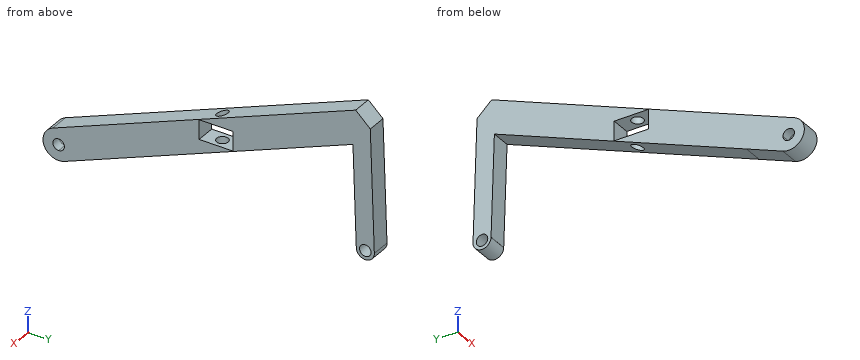
```python
from build123d import *

# Parameters (mm, degrees)
BOSS_EXTRUDE1_DEPTH     = 2.54
SKETCH2_W               = 5.08
SKETCH2_H               = 8.89
CUT_EXTRUDE1_DEPTH      = 5.08
CUT_EXTRUDE2_DEPTH      = 86.150645665
CUT_EXTRUDE2_DEPTH_BACK = 86.150645665
SKETCH3_R               = 1.5


with BuildPart() as part:
    # Sketch1 → Boss-Extrude1 (new, symmetric)
    with BuildSketch(Plane(origin=(0, 0, 0), x_dir=(0, 0, -1), z_dir=(1, 0, 0))):
        with BuildLine():
            ThreePointArc((-3.792924612, -1.516297351), (1.516297351, -3.792924612), (3.792924612, 1.516297351))
            Line((3.792924612, 1.516297351), (0, 11.004065103))
            Line((0, 11.004065103), (-26.293066659, 76.774555024))
            Line((-26.293066659, 76.774555024), (0, 77.645444775))
            Line((0, 77.645444775), (0, 77.657240774))
            Line((0, 77.657240774), (0.077903078, 77.648025113))
            ThreePointArc((0.077903078, 77.648025113), (2.351974887, 80.077903078), (-0.077903078, 82.351974887))
            Line((-0.077903078, 82.351974887), (-31.810501027, 81.300914746))
            Line((-31.810501027, 81.300914746), (-35.377927791, 77.491646464))
            Line((-35.377927791, 77.491646464), (-3.792924612, -1.516297351))
        make_face()
        with BuildLine():
            ThreePointArc((1.5, 0), (-1.060660172, -1.060660172), (0, 1.5))
            ThreePointArc((0, 1.5), (1.060660172, 1.060660172), (1.5, 0))
        make_face(mode=Mode.SUBTRACT)
        with BuildLine():
            ThreePointArc((1.5, 80), (1.060660172, 78.939339828), (0, 78.5))
            ThreePointArc((0, 78.5), (-1.060660172, 81.060660172), (1.5, 80))
        make_face(mode=Mode.SUBTRACT)
    extrude(amount=BOSS_EXTRUDE1_DEPTH, both=True)

    # Sketch2 → Cut-Extrude1 (cut)
    with BuildSketch(Plane(origin=(2.54, 0, 0), x_dir=(0, 0, -1), z_dir=(1, 0, 0))):
        with Locations((-16.420936138, 41.075962298)):
            Rectangle(SKETCH2_W, SKETCH2_H)
    extrude(amount=-CUT_EXTRUDE1_DEPTH, mode=Mode.SUBTRACT)

    # Sketch3 → Cut-Extrude2 (cut, two sides: drawn at the far end of the back side and taken through both)
    with BuildSketch(Plane.XY.offset(13.880936138).offset(-CUT_EXTRUDE2_DEPTH_BACK)):
        with Locations(Location((0, 41.075962298, 0), (0, 0, 90))):
            Circle(SKETCH3_R)
    extrude(amount=CUT_EXTRUDE2_DEPTH + CUT_EXTRUDE2_DEPTH_BACK, mode=Mode.SUBTRACT)


solid = part.part
```
Input: part model. Units: mm. Frame: model coordinates. Round coordinates to 2 decimals unless told otherwise and drop trailing zeros. Loops run counter-clockwise (first coordinate to the right, second up) from the corner with the lowest first, then second, coordinate; pieces in that order, holes last. Notation, with made-up numbers: (20, -16) -> (67, -16) arc R23 ccw to (67, -2) -> close; hole circle Ø8 at (-29.5, 61). An arc over 180 degrees is marked (long way). Use one line per item in the form item = value. Start each with the question number.
Item 1: Contact query for flat-ended pins moving along their axis: pin 1 Ø1.5 at (x, z) = (-1.5, 26.5) entering from +Y; pin 2 Ø2.5 at (x, z) = (-0.5, 17) entering from +Y; pin 3 Ø1.5 at (x, y) = (0, 40) entering from +Z; pin 4 Ø4 at (y, z) = (0, 0) entering from +X. Output: stop coordinate, or through.
Item 2: Material intervals for L1, parallel to Z at x = 1.2, y = 0; L2, parallel to Z at x = -2.3, y = 37.5; L3, parallel to Z at x = -1.1, y = 71, sorted ascending. Write a range as from..to.
Item 3: Section query D-D on y = 20.5. Return the cut outline in (x, z), then the cut area to 3 significant figures.
Item 4: Section query B-B on y = 80. Return the cut outline in (x, z).
Item 5: Section query A-A on y = 44.5. Return the cut outline in (x, z).
Item 6: Section query C-C on z = 31. Return the cut outline in (x, y), then the cut area to 3 significant figures.
Ans:
q1.pin_1 = 81.5
q1.pin_2 = 81.83
q1.pin_3 = 20.29
q1.pin_4 = 2.54
q2.L1 = -4.08..-1.5, 1.5..4.4
q2.L2 = 10.59..13.88, 18.96..19.39
q2.L3 = 23.98..32.78
q3.outline = (-2.54, 3.8) -> (2.54, 3.8) -> (2.54, 12.59) -> (-2.54, 12.59) -> close
q3.area = 44.7 mm^2
q4.outline = (-2.54, -2.35) -> (2.54, -2.35) -> (2.54, -1.5) -> (-2.54, -1.5) -> close; (-2.54, 1.5) -> (2.54, 1.5) -> (2.54, 33.03) -> (-2.54, 33.03) -> close
q5.outline = (-2.54, 13.39) -> (2.54, 13.39) -> (2.54, 13.88) -> (-2.54, 13.88) -> close; (-2.54, 18.96) -> (2.54, 18.96) -> (2.54, 22.19) -> (-2.54, 22.19) -> close
q6.outline = (-2.54, 66.54) -> (2.54, 66.54) -> (2.54, 81.33) -> (-2.54, 81.33) -> close
q6.area = 75.1 mm^2
